```python
from build123d import *

# Parameters (mm, degrees)
EXTRUDE_START         = 7
SKETCH_1_R            = 40
SKETCH_1_R_2          = 9
EXTRUDE_1_DEPTH       = 13
SKETCH_12_R           = 43.016285751
SKETCH_12_R_2         = 18
CUT_EXTRUDE_5_DEPTH   = 7
CUT_EXTRUDE_5_2_DEPTH = 10
EXTRUDE_START_2       = -8
SKETCH_17_R           = 9
SKETCH_17_R_2         = 3.5
EXTRUDE_6_DEPTH       = 8
FILLET_1_R            = 7


with BuildPart() as part:
    # Эскиз1 → Вытянуть1 (new body)
    with BuildSketch(Plane(origin=(0, 0, 0), x_dir=(1, 0, 0), z_dir=(0, 1, 0)).offset(EXTRUDE_START)):
        with Locations(Location((0, 0, 0), (0, 0, 90))):
            Circle(SKETCH_1_R)
        with Locations(Location((0, 0, 0), (0, 0, 90))):
            Circle(SKETCH_1_R_2, mode=Mode.SUBTRACT)
    extrude(amount=EXTRUDE_1_DEPTH)

    # Эскиз12 → Cut-Extrude 5 (cut)
    with BuildSketch(Plane.XZ.offset(-7)):
        Circle(SKETCH_12_R)
        with Locations(Location((0, 0, 0), (0, 0, 270))):
            Circle(SKETCH_12_R_2, mode=Mode.SUBTRACT)
    extrude(amount=-CUT_EXTRUDE_5_DEPTH, mode=Mode.SUBTRACT)

    # Эскиз16 → Cut-Extrude 5 2 (cut)
    with BuildSketch(Plane(origin=(0, 20, 0), x_dir=(1, 0, 0), z_dir=(0, 1, 0))):
        Polygon((-7.191454283, -44.519977242), (-37.881198424, -24.469576927), (-45.366952085, 5.371359597), (-23.143023154, 39.387971833), (7.640311576, 44.595915214), (37.770432201, 24.911131357), (46.151265064, -5.857681321), (23.11557492, -39.392615521), align=None)
        Polygon((-8.732909884, 36.547470459), (12.235760297, 37.752192063), (31.649059452, 24.416882045), (39.477467189, -1.213541002), (15.512644169, -36.101089761), (-9.76688891, -38.545852744), (-32.285837438, -23.077221806), (-37.797558071, -5.764310018), align=None, mode=Mode.SUBTRACT)
    extrude(amount=-CUT_EXTRUDE_5_2_DEPTH, mode=Mode.SUBTRACT)

    # Эскиз17 → Вытянуть6 (add)
    with BuildSketch(Plane(origin=(0, 20, 0), x_dir=(1, 0, 0), z_dir=(0, 1, 0)).offset(EXTRUDE_START_2)):
        with Locations(Location((0, 0, 0), (0, 0, 90))):
            Circle(SKETCH_17_R)
        with Locations(Location((0, 0, 0), (0, 0, 270))):
            Circle(SKETCH_17_R_2, mode=Mode.SUBTRACT)
    extrude(amount=EXTRUDE_6_DEPTH)

    # Скругление1
    fillet_1_edges = [part.edges().sort_by_distance(p)[0] for p in [
        (0, 14, 18),
    ]]
    fillet(fillet_1_edges, radius=FILLET_1_R - 0.0001)  # a hair under: the kernel refuses the full size


solid = part.part
```
Verification items for the finished model (mm, model axes). A direction names the side the tool comes from. Give positions to 0.01 mm unless a question says otherwise; leave off trailing zeros. Loops run counter-clockwise (first coordinate to the right, second up) from the corner with the lowest first, then second, coordinate; pieces in that order, holes last.
1. Thickness scan on line 1 (X direction, y = 9.7, z = 0); line 2 (Y direction, x = 19, z = -22.5); line 3 (Y direction, x = 4.5, z = 7.5). Record the ranges inside material, lowest first.
2. Set-up check for faces 1 (the flat face through (3.05, 17.042, 37.306)), 2 (the flat face through (4, 12, 0)): record each of +Z, -Z, +X, -X, +Y, -Y from which the full face is reachable in a straight line by a thin tool's end or side.
3. Mould release check, pull along X, two halves, no side actions. Record for faces 3 (the flat face through (27.663, 17.042, 18.413)), 4 (the cylindrical face through (-3.417, 15.944, -0.759)), 5 (the flat face through (26, 14, 1)): released by +X, released by -X, zero draft, split by the parting line, or undercut.
4. Section check A-A, the plane y = 16. Enter the section's corners in (x, z), then the cut area to 3 significant figures.
5. Section check D-D, the plane z = 27.5. Enter the section's corners in (x, y).
6. Go/stop test with flat-tipped pins: pin 1 Ø1.5 at (y, z) = (17.5, -4) entering from -X; pin 2 Ø14.5 at (x, z) = (0, 0) entering from -Y; pin 3 Ø1 at (x, y) = (-10.5, 18.5) entering from +Z. Record where each tip stops, or that it passes through.
Geometry says:
1. line 1: x = -18.54 to -9, 9 to 18.54
1. line 2: y = 14 to 20
1. line 3: y = 12 to 20
2. face 1: +Z, +X, +Y, -Y
2. face 2: -Y
3. face 3: released by +X
3. face 4: undercut
3. face 5: zero draft
4. outline: (-37.8, 5.76) - (-8.73, -36.55) - (12.24, -37.75) - (31.65, -24.42) - (39.48, 1.21) - (15.51, 36.1) - (-9.77, 38.55) - (-32.29, 23.08) - close; hole circle Ø7 at (0, 0)
4. area: 4,050 mm2
5. outline: (-25.85, 14) - (21.42, 14) - (21.42, 20) - (-25.85, 20) - close
6. pin 1: stops at x = -31.61
6. pin 2: stops at y = 12
6. pin 3: stops at z = 38.39
